from build123d import *

# Parameters (mm, degrees)
F0_R        = 6
F1_DEPTH    = 135
F3_START    = -2
F3_DEPTH    = 4.0010001005
F4_START    = 2
F4_DEPTH    = 4
F5_T2_ANGLE = 325.4889919963
F5_T4_ANGLE = 306.0016128171
F5_T6_ANGLE = 306.0016128171
F6_R        = 2
F7_DEPTH    = 12.5
F8_R        = 4.8
F9_DEPTH    = 6
F10_R       = 2.375
F11_DEPTH   = 7.5


# Not quite as in the source:
# - a fillet or chamfer that OpenCascade refuses, or shapes differently, is made with other operations: its cross-section is extruded or revolved along the edge and cut away or added


with BuildPart() as f1:
    # F0 (on Top) → F1 (new body)
    with BuildSketch(Plane.XY):
        Circle(F0_R)
    extrude(amount=F1_DEPTH)

    # F2 (on Front) → F3 (cut)
    with BuildSketch(Plane.XZ.offset(F3_START)):
        with BuildLine():
            Line((-6.0225790367, 135.0244730711), (-6.0225790367, 124.5302637944))
            ThreePointArc((-6.0225790367, 124.5302637944), (0.1221735447, 121.5009951577), (6.1649857089, 124.7288232056))
            Line((6.1649857089, 124.7288232056), (6.1649857089, 135.0244730711))
            Line((6.1649857089, 135.0244730711), (-6.0225790367, 135.0244730711))
        make_face()
    extrude(amount=-F3_DEPTH, mode=Mode.SUBTRACT)

    # F2 (on Front) → F4 (cut)
    with BuildSketch(Plane.XZ.offset(F4_START)):
        with BuildLine():
            Line((-6.0225790367, 135.0244730711), (-6.0225790367, 124.5302637944))
            ThreePointArc((-6.0225790367, 124.5302637944), (0.1221735447, 121.5009951577), (6.1649857089, 124.7288232056))
            Line((6.1649857089, 124.7288232056), (6.1649857089, 135.0244730711))
            Line((6.1649857089, 135.0244730711), (-6.0225790367, 135.0244730711))
        make_face()
    extrude(amount=F4_DEPTH, mode=Mode.SUBTRACT)

    # F5: fillet of radius 6 on 3 edges, made by hand

    # F5_s1 → F5_t2 (revolve, cut)
    with BuildSketch(Plane(origin=(0, 0, 0), x_dir=(0, 0, 1), z_dir=(0.2966333156, -0.9549914534, 0))):
        with BuildLine():
            ThreePointArc((128.9990343146, -6.0004), (133.242299252, -4.2429820947), (135.0003999223, 0))
            Line((135.0003999223, 0), (135.6005365042, 0))
            Line((135.6005365042, 0), (135.6001365685, -6))
            Line((135.6001365685, -6), (135, -6.6001365685))
            ThreePointArc((135, -6.6001365685), (131.9995171573, -6.6001365685), (128.9990343146, -6.6005365685))
            Line((128.9990343146, -6.6005365685), (128.9990343146, -6.0004))
        make_face()
    revolve(axis=Axis((0, 0, 135), (0, 0, 1)), revolution_arc=F5_T2_ANGLE, mode=Mode.SUBTRACT)

    # F5_s3 → F5_t4 (revolve, cut)
    with BuildSketch(Plane(origin=(0, 0, 0), x_dir=(0, 0, 1), z_dir=(-0.5981120695, 0.8014124733, 0))):
        with BuildLine():
            ThreePointArc((128.9990343146, -6.0004), (133.242299252, -4.2429820947), (135.0003999223, 0))
            Line((135.0003999223, 0), (135.6005365042, 0))
            Line((135.6005365042, 0), (135.6001365685, -6))
            Line((135.6001365685, -6), (135, -6.6001365685))
            ThreePointArc((135, -6.6001365685), (131.9995171573, -6.6001365685), (128.9990343146, -6.6005365685))
            Line((128.9990343146, -6.6005365685), (128.9990343146, -6.0004))
        make_face()
    revolve(axis=Axis((0, 0, 135), (0, 0, 1)), revolution_arc=F5_T4_ANGLE, mode=Mode.SUBTRACT)

    # F5_s5 → F5_t6 (revolve, cut)
    with BuildSketch(Plane(origin=(0, 0, 0), x_dir=(0, 0, 1), z_dir=(-0.2967679759, 0.9549496157, 0))):
        with BuildLine():
            ThreePointArc((128.9990343146, -6.0004), (133.242299252, -4.2429820947), (135.0003999223, 0))
            Line((135.0003999223, 0), (135.6005365042, 0))
            Line((135.6005365042, 0), (135.6001365685, -6))
            Line((135.6001365685, -6), (135, -6.6001365685))
            ThreePointArc((135, -6.6001365685), (131.9995171573, -6.6001365685), (128.9990343146, -6.6005365685))
            Line((128.9990343146, -6.6005365685), (128.9990343146, -6.0004))
        make_face()
    revolve(axis=Axis((0, 0, 135), (0, 0, 1)), revolution_arc=F5_T6_ANGLE, mode=Mode.SUBTRACT)

    # F6 (on face) → F7 (cut, symmetric)
    with BuildSketch(Plane.XZ):
        with Locations((0, 129)):
            Circle(F6_R)
    extrude(amount=F7_DEPTH, both=True, mode=Mode.SUBTRACT)

    # F8 (on face) → F9 (cut)
    with BuildSketch(Plane(origin=(0, 0, 0), x_dir=(1, 0, 0), z_dir=(0, 0, -1))):
        Circle(F8_R)
    extrude(amount=-F9_DEPTH, mode=Mode.SUBTRACT)

    # F10 (on face) → F11 (join)
    with BuildSketch(Plane(origin=(0, 0, 6), x_dir=(1, 0, 0), z_dir=(0, 0, -1))):
        Circle(F10_R)
    extrude(amount=F11_DEPTH)


solid = f1.part
Input: part model. Units: mm. Frame: model coordinates. A direction names the side the tool comes from. Give positions to 0.01 mm unless a question says otherwise; leave off trailing zeros. Loops run counter-clockwise (first coordinate to the right, second up) from the corner with the lowest first, then second, coordinate; pieces in that order, holes last. Notation, with made-up numbers: (50.5, -18) - (64.5, -18) arc R29 cw to (64.5, 5) - close; hole circle Ø5 at (-25.5, 30). An arc over 180 degrees is marked (long way). Use CSV: the item, a comma, the result in double quotes. Start each with the question number.
Item 1: Section A-A on z = 75. Return loops of the section in (x, y), then the cut area to 3 significant figures.
Item 2: Mould query, pull axis Y, two halves, no side actions, for faces 5 (the flat face through (2, 2, 6)), 6 (the flat face through (0, 0, -1.5)), 7 (the flat face through (-0.1, 2, 126.7)). Classes: pulls with the +Y half, pulls with the -Y half, needs draft (parallel to the pull), parting line crosses it, or undercut.
Item 3: Reachability of faces 1 (the cylindrical face through (-0.1, 3.5, 121.5)), 2 (the cylindrical face through (-0.1, -3.5, 121.5)), 3 (the flat face through (-3, 4, 0)), 4 (the cylindrical face through (0, 0, 131)) from +Z, -Z, +X, -X, +Y, -Y: full face, straight path, thin tool, end or side. Return the list, or none.
Item 4: Contact query for flat-ended pins moving along their axis: P1, Ø1.5, axis at y = 4.5, z = 23.5, coming from the +X side; P2, Ø5.5, axis at x = -1, z = 129.5, coming from the +Y side; P3, Ø1.5, axis at x = 1.5, y = 0.5, coming from the +Z side. Output: stop coordinate, or through.
Item 5: Line query: line 1 (Y direction, x = 0, z = 4.6) (3 decimals); line 2 (X direction, y = 0.3, z = 129). Output: solid intervals per line, ascending.
Ans:
1,outline,"circle Ø12 at (0, 0)"
1,area,"113 mm2"
2,face 5,"undercut"
2,face 6,"needs draft"
2,face 7,"pulls with the +Y half"
3,face 1,"+Z, +Y"
3,face 2,"+Z, -Y"
3,face 3,"-Z"
3,face 4,"+Y, -Y"
4,P1,"stops at x = 4.68"
4,P2,"stops at y = 2"
4,P3,"stops at z = 134.94"
5,line 1,"y = -6 to -4.8, -2.375 to 2.375, 4.8 to 6"
5,line 2,"x = -5.99 to -2, 2 to 5.99"
